Autodesk Inventor part; units mm, degrees
ref_plane "YZ Plane" through (0, 0, 0) normal (1, 0, 0) x (0, 1, 0)
ref_plane "XZ Plane" through (0, 0, 0) normal (0, 1, 0) x (-1, 0, 0)
ref_plane "XY Plane" through (0, 0, 0) normal (0, 0, 1) x (1, 0, 0)
sketch "Boceto1" plane through (0, 0, 0) normal (0, 1, 0) x (-1, 0, 0)
  line L0 (34.5, 0) -> (34.5, 24)
  line L1 (34.5, 24) -> (47.5, 24)
  line L2 (24, 47.5) -> (24, 34.5)
  line L3 (24, 34.5) -> (-24, 34.5)
  line L4 (-24, 34.5) -> (-24, 47.5)
  line L5 (-34.5, 24) -> (-47.5, 24)
  line L6 (47.5, 0) -> (-47.5, 0) construction
  line L7 (-47.5, 47.5) -> (-24, 47.5)
  line L8 (24, 47.5) -> (47.5, 47.5)
  line L9 (-47.5, 24) -> (-47.5, 47.5)
  line L10 (47.5, 47.5) -> (47.5, 24)
  line L11 (-34.5, 24) -> (-34.5, 0)
  line L12 (34.5, 0) -> (34.5, -24)
  line L13 (34.5, -24) -> (47.5, -24)
  line L14 (24, -47.5) -> (24, -34.5)
  line L15 (24, -34.5) -> (-24, -34.5)
  line L16 (-24, -34.5) -> (-24, -47.5)
  line L17 (-34.5, -24) -> (-47.5, -24)
  line L18 (-47.5, -47.5) -> (-24, -47.5)
  line L19 (24, -47.5) -> (47.5, -47.5)
  line L20 (-47.5, -24) -> (-47.5, -47.5)
  line L21 (47.5, -47.5) -> (47.5, -24)
  line L22 (-34.5, -24) -> (-34.5, 0)
  line L23 (-47.5, -47.5) -> (47.5, 47.5) construction
  line L24 (-47.5, 47.5) -> (47.5, -47.5) construction
  point P0 (0, 0)
  point P1 (0, -34.5)
  point P2 (24, 41)
  point P3 (0, 0)
  point P4 (35.75, 47.5)
  dimension "d0" = 95
  dimension "d9" = 13
  dimension "d10" = 23.5
  dimension "d15" = 23.5
  dimension "d71" = 95
extrude "Extrusión1" add sketch "Boceto1" along normal blind 7
chamfer "Chaflán4" distance 3.2 angle 45 4 edges at (24, 3.5, 34.5) (34.5, 3.5, 24) (-24, 3.5, -34.5) (-34.5, 3.5, -24)
sketch "Boceto2" plane through (0, 7, 0) normal (0, 1, 0) x (1, 0, 0)
  line L0 (-27.5, -27.5) -> (27.5, -27.5)
  line L1 (27.5, -27.5) -> (27.5, 27.5)
  line L2 (27.5, 27.5) -> (-27.5, 27.5)
  line L3 (-27.5, 27.5) -> (-27.5, -27.5)
  line L4 (-27.5, -27.5) -> (27.5, 27.5) construction
  line L5 (27.5, -27.5) -> (-27.5, 27.5) construction
  line L6 (-29.9749, 18.6612) -> (-18.6612, 29.9749)
  line L7 (-18.6612, 29.9749) -> (-25.0251, 36.3388)
  line L8 (-25.0251, 36.3388) -> (-36.3388, 25.0251)
  line L9 (-36.3388, 25.0251) -> (-29.9749, 18.6612)
  line L10 (-29.9749, 18.6612) -> (-25.0251, 36.3388) construction
  line L11 (-18.6612, 29.9749) -> (-36.3388, 25.0251) construction
  line L12 (-15.4792, 28.2071) -> (-26.7929, 39.5208)
  line L13 (-26.7929, 39.5208) -> (-39.5208, 26.7929)
  line L14 (-39.5208, 26.7929) -> (-28.2071, 15.4792)
  line L15 (-28.2071, 15.4792) -> (-15.4792, 28.2071)
  line L16 (-15.4792, 28.2071) -> (-39.5208, 26.7929) construction
  line L17 (-26.7929, 39.5208) -> (-28.2071, 15.4792) construction
  line L18 (-34.5, 24) -> (-34.5, -24)
  line L19 (-34.5, 0) -> (34.5, 0) construction
  line L20 (34.5, -24) -> (34.5, 24)
  line L21 (-18.6612, 29.9749) -> (-15.4792, 28.2071)
  line L22 (-29.9749, 18.6612) -> (-28.2071, 15.4792)
  line L23 (29.9749, -18.6612) -> (18.6612, -29.9749)
  line L24 (18.6612, -29.9749) -> (36.3388, -25.0251) construction
  line L25 (18.6612, -29.9749) -> (15.4792, -28.2071)
  line L26 (15.4792, -28.2071) -> (39.5208, -26.7929) construction
  line L27 (25.0251, -36.3388) -> (36.3388, -25.0251)
  line L28 (29.9749, -18.6612) -> (25.0251, -36.3388) construction
  line L29 (18.6612, -29.9749) -> (25.0251, -36.3388)
  line L30 (26.7929, -39.5208) -> (28.2071, -15.4792) construction
  line L31 (15.4792, -28.2071) -> (26.7929, -39.5208)
  line L32 (26.7929, -39.5208) -> (39.5208, -26.7929)
  line L33 (28.2071, -15.4792) -> (15.4792, -28.2071)
  line L34 (36.3388, -25.0251) -> (29.9749, -18.6612)
  line L35 (29.9749, -18.6612) -> (28.2071, -15.4792)
  line L36 (39.5208, -26.7929) -> (28.2071, -15.4792)
  point P0 (0, 0)
  point P1 (-27.5, 27.5)
  point P2 (27.5, -27.5)
  point P3 (27.5, -27.5)
  point P4 (34.5, -24)
  dimension "d21" = 55
  dimension "d22" = 55
  dimension "d23" = 16
  dimension "d24" = 9
  dimension "d25" = 18
  dimension "d26" = 16
  dimension "d51" = 135
  dimension "d52" = 135
  dimension "d55" = 360
sketch "Boceto3" plane through (0, 0, 0) normal (0, -1, 0) x (1, 0, 0)
  line L0 (47.5, 47.5) -> (47.5, 24)
  line L1 (47.5, 47.5) -> (24, 47.5)
  line L2 (24, 47.5) -> (24, 24)
  line L3 (24, 24) -> (47.5, 24)
  line L4 (47.5, 24) -> (47.5, 47.5)
  line L5 (24, 34.5) -> (24, 47.5)
  line L6 (47.5, 24) -> (34.5, 24)
  circle A0 centre (40.75, 40.75) radius 2.5
  line L7 (0, 48.9307) -> (0, -48.9307) construction
  line L8 (51.06, 0) -> (-51.06, 0) construction
  circle A1 centre (-40.75, 40.75) radius 2.5
  circle A2 centre (-40.75, -40.75) radius 2.5
  circle A3 centre (40.75, -40.75) radius 2.5
  line L9 (47.5, 47.5) -> (24, 24) construction
  line L10 (24, 47.5) -> (47.5, 24) construction
  point P0 (0, 0)
  point P1 (0, 0)
  point P2 (35.75, 35.75)
  dimension "d41" = 5
  dimension "d77" = 360
  dimension "d80" = 5
extrude "Extrusión6" cut sketch "Boceto3" against normal blind 4 contours A0 | A1 | A2 | A3
sketch "Boceto4" plane through (0, 7, 0) normal (0, 1, 0) x (1, 0, 0)
  circle A0 centre (0, 0) radius 3.3
  dimension "d44" = 6.6
extrude "Extrusión7" cut sketch "Boceto4" against normal up to next
sketch "Boceto5" plane through (0, 0, 0) normal (0, -1, 0) x (1, 0, 0)
  circle A0 centre (0, 0) radius 6.5
  dimension "d47" = 13
extrude "Extrusión8" cut sketch "Boceto5" against normal blind 4
extrude "Extrusión9" add sketch "Boceto2" along normal blind 4 contours L25 L29 L27 L34 L20 L36 L32 L31 | L14 L18 L9 L22 | L36 L20 L34 L35 | L14 L13 L12 L21 L7 L8 L9 L18
extrude "Extrusión10" add sketch "Boceto2" along normal blind 2 contours L33 L1 L23 L0 | L0 L23 L25 L33 | L15 L22 L6 L3 | L3 L6 L2 L15 | L33 L35 L23 L1 | L2 L6 L21 L15
chamfer "Chaflán3" distance 2 angle 45 4 edges at (-17.0702, 9, -29.091) (-29.091, 9, -17.0702) (29.091, 9, 17.0702) (17.0702, 9, 29.091)
sketch "Boceto7" plane through (0, 7, 0) normal (0, 1, 0) x (1, 0, 0)
  line L0 (20.7825, -32.0962) -> (32.0962, -20.7825)
  line L1 (32.0962, -20.7825) -> (29.9749, -18.6612)
  line L2 (29.9749, -18.6612) -> (18.6612, -29.9749)
  line L3 (18.6612, -29.9749) -> (20.7825, -32.0962)
  line L4 (20.7825, -32.0962) -> (29.9749, -18.6612) construction
  line L5 (32.0962, -20.7825) -> (18.6612, -29.9749) construction
  line L6 (20.132, -28.5041) -> (28.5041, -20.132)
  line L7 (18.6612, -29.9749) -> (25.0251, -36.3388)
  line L8 (-20.7825, 32.0962) -> (-32.0962, 20.7825)
  line L9 (-32.0962, 20.7825) -> (-29.9749, 18.6612)
  line L10 (-29.9749, 18.6612) -> (-18.6612, 29.9749)
  line L11 (-18.6612, 29.9749) -> (-20.7825, 32.0962)
  line L12 (-20.7825, 32.0962) -> (-29.9749, 18.6612) construction
  line L13 (-32.0962, 20.7825) -> (-18.6612, 29.9749) construction
  line L14 (36.3388, -25.0251) -> (29.9749, -18.6612)
  point P0 (0, 0)
  point P1 (25.3787, -25.3787)
  point P2 (-20.132, 28.5041)
  point P3 (-28.5041, 20.132)
  point P4 (-18.6612, 29.9749)
  point P5 (-25.3787, 25.3787)
  point P6 (33.5, -22.1863)
  dimension "d64" = 3
  dimension "d67" = 360
extrude "Extrusión11" cut sketch "Boceto7" against normal up to next
fillet "Empalme1" radius 3 16 edges at (24, 3.5, 47.5) (47.5, 3.5, 47.5) (47.5, 3.5, 24) (47.5, 3.5, -24) (34.5, 3.5, -24) (47.5, 3.5, -47.5) (24, 3.5, -47.5) (24, 3.5, -34.5) (-24, 3.5, -47.5) (-47.5, 3.5, -47.5) (-47.5, 3.5, -24) (-47.5, 3.5, 24) (-34.5, 3.5, 24) (-47.5, 3.5, 47.5) (-24, 3.5, 47.5) (-24, 3.5, 34.5)
equation "\"d15\" = d13"
properties part number "SistemaDeDesacople"
Could you check a few things on this model? Use its own coordinates, in mm. A direction names the side the tool comes from. Round coordinates to 2 decimals unless told otherwise and drop trailing zeros. Write each loop counter-clockwise with the first axis right and the second up, starting at its lowest first coordinate (ties: lowest second). Pieces come first, ordered by that corner, then holes. Notation, with made-up numbers: (20.5, -12.75) - (38.5, -12.75) arc R22 ccw to (38.5, 17.25) - close; hole circle Ø10 at (-26.5, -20). An arc over 180 degrees is marked (long way). Use a Markdown table: item, result.
Q1. Thinking about a two-plate mould opening in Z: for faces 5 (the cylindrical face through (24.9, 3.55, -46.64)), 6 (the flat face through (-28, 7, -28)), 7 (the flat face through (24, 3, 41)), which applies, released by +Z, released by -Z, zero draft, split by the parting line, or undercut?
Output values:
| item | result |
|---|---|
| face 5 | released by -Z |
| face 6 | undercut |
| face 7 | zero draft |
Q2. I want a section at D-D (z = 40.75). List the corners of the cut face in (x, y) for me, plus the area to 3 significant figures.
Output values:
| item | result |
|---|---|
| outline | (-47.5, 0) - (-43.25, 0) - (-43.25, 4) - (-38.25, 4) - (-38.25, 0) - (-24, 0) - (-24, 7) - (-47.5, 7) - close; (24, 0) - (38.25, 0) - (38.25, 4) - (43.25, 4) - (43.25, 0) - (47.5, 0) - (47.5, 7) - (24, 7) - close |
| area | 289 mm2 |
Q3. I want a section at B-B (z = 0). List the corners of the cut face in (x, y) for me, plus the area to 3 significant figures.
Output values:
| item | result |
|---|---|
| outline | (-34.5, 0) - (-6.5, 0) - (-6.5, 4) - (-3.3, 4) - (-3.3, 7) - (-34.5, 7) - close; (3.3, 4) - (6.5, 4) - (6.5, 0) - (34.5, 0) - (34.5, 7) - (3.3, 7) - close |
| area | 411 mm2 |
Q4. I want a section at C-C (x = 0). List the corners of the cut face in (y, z) for me.
Output values:
| item | result |
|---|---|
| outline | (0, -34.5) - (7, -34.5) - (7, -3.3) - (4, -3.3) - (4, -6.5) - (0, -6.5) - close; (0, 6.5) - (4, 6.5) - (4, 3.3) - (7, 3.3) - (7, 34.5) - (0, 34.5) - close |
Q5. For faces 1 (the flat face through (26.36, 3.55, 26.52)), 2 (the flat face through (41, 4, 41)), 3 (the flat face through (28.329, 9.986, 17.786)), 4 (the flat face through (21.932, 8.083, 21.754)), which set-ups out of +Z, -Z, +X, -X, +Y, -Y let a thin tool reach every point of the face, with its end or its side?
Output values:
| item | result |
|---|---|
| face 1 | +Y, -Y |
| face 2 | -Y |
| face 3 | -X, +Y |
| face 4 | -Z, -X, +Y |
Q6. Please list where these lines run through material, in increasing order: L1, parallel to Z at x = 41, y = 2.5; L2, parallel to X at y = 6.5, z = 40.5; L3, parallel to Z at x = 0, y = 1.35.
Output values:
| item | result |
|---|---|
| L1 | -47.5 to -43.24, -38.26 to -24, 24 to 38.26, 43.24 to 47.5 |
| L2 | -47.5 to -24, 24 to 47.5 |
| L3 | -34.5 to -6.5, 6.5 to 34.5 |
Q7. I want a section at A-A (x = 40.75). List the corners of the cut face in (y, z) for me, plus the area to 3 significant figures.
Output values:
| item | result |
|---|---|
| outline | (0, -47.5) - (7, -47.5) - (7, -24) - (0, -24) - (0, -38.25) - (4, -38.25) - (4, -43.25) - (0, -43.25) - close; (0, 24) - (7, 24) - (7, 47.5) - (0, 47.5) - (0, 43.25) - (4, 43.25) - (4, 38.25) - (0, 38.25) - close |
| area | 289 mm2 |
Q8. For pin 1 (5.5 mm diameter, centred on x = 40, z = 42, fed in from -Y); pin 2 (3 mm diameter, centred on x = -40.75, z = 40.75, fed in from +Y); pin 3 (4 mm diameter, centred on y = 2, z = 18.5, fed in from -X); pin 4 (4.5 mm diameter, centred on x = -40.75, z = -40.75, fed in from -Y), each with a flat end and sliding along its axis, tell me the tip position at first contact or that it passes through.
Output values:
| item | result |
|---|---|
| pin 1 | y = 0 |
| pin 2 | y = 7 |
| pin 3 | x = -34.5 |
| pin 4 | y = 4 |
